Answer from the drawing. Dimensions are ordinates in mm from the lowest x, y and z of the part. A direction names the side the tool comes from. Coordinates: 2 decimals unless noted, no trailing zeros. Order: outer loops, then holes, each group sorted by start corner. A loop starts at its lowest first (then second) coordinate and runs counter-clockwise, first axis right, second up. Notation, with made-up numbers: M 78.25,5 L 95.25,5 A16 cw 95.25,32 Z; hole C 34,70.25 d8. An arc over 180 degrees is marked long. One line per question, with ' | ' between items. Start each with the question number.
1) Find section A-A, the plane z = 12. Write down the section's boundary in (x, y).
2) Find section D-D, the plane x = 24. Write down the section's boundary in (y, z), plus the area to 3 significant figures.
3) Find section B-B, the plane x = 2. Write down the section's boundary in (y, z).
4) Consider probe 1 along Z at (x, y) = (3, 5); probe 2 along Y at (x, z) = (10.75, 5.5); probe 3 along X at (y, z) = (62.5, 11). Determine where each line is inside the solid, lowest interval first.
5) The mould has two halves that part along Y. Classify the marked faces 1, 2 and 3: +Y half, -Y half, draft (parallel to the pull), parting line (faces both ways), or undercut.
6) Given P1, Ø5, axis at y = 61.5, z = 7.5, coming from the -X side; P2, Ø6, axis at y = 23, z = 7.5, coming from the -X side; P3, Ø1, axis at y = 8, z = 15.5, coming from the -X side; P4, Ø5, axis at y = 58, z = 14, coming from the +X side, each flat-ended and moving along its own axis, determine where each tip first touches the part or whether it passes through.
7) Find section C-C, the plane y = 58.5. Write down the section's boundary in (x, z), plus the area to 3 significant figures.
8) A tool of negligible diameter and unlimited length cuts with its end or side. For the marked faces 4, 5 and 6, from which of +Z, -Z, +X, -X, +Y, -Y can it reach the whole face along a straight path? Write none if from no direction.
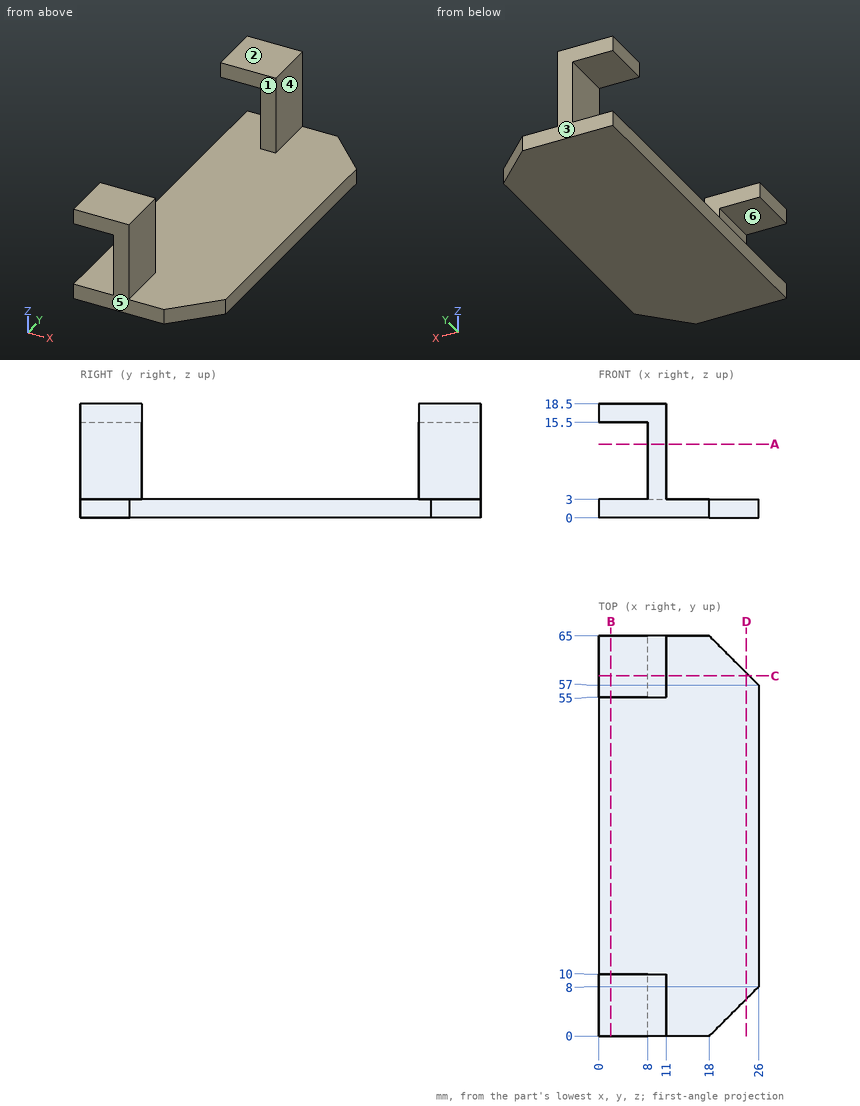
Report:
1) outline: M 8,0 L 11,0 L 11,10 L 8,10 Z; M 8,55 L 11,55 L 11,65 L 8,65 Z
2) outline: M 6,0 L 59,0 L 59,3 L 6,3 Z | area: 159 mm^2
3) outline: M 0,0 L 65,0 L 65,3 L 0,3 Z; M 0,15.5 L 10,15.5 L 10,18.5 L 0,18.5 Z; M 55,15.5 L 65,15.5 L 65,18.5 L 55,18.5 Z
4) probe 1: z = 0 to 3, 15.5 to 18.5 | probe 2: y = 0 to 10, 55 to 65 | probe 3: x = 8 to 11
5) face 1: undercut | face 2: draft | face 3: +Y half
6) P1: stops at x = 8 | P2: passes through | P3: stops at x = 0 | P4: stops at x = 11
7) outline: M 0,0 L 24.5,0 L 24.5,3 L 11,3 L 11,18.5 L 0,18.5 L 0,15.5 L 8,15.5 L 8,3 L 0,3 Z | area: 144 mm^2
8) face 4: +Z, +X, +Y, -Y | face 5: +Z, -Z, +X, -X, -Y | face 6: -X, +Y, -Y
